```python
from build123d import *

# Parameters (mm, degrees)
F0_R     = 3.1
F1_DEPTH = 10
F2_DEPTH = 1.5
F3_W     = 10
F3_H     = 2
F4_DEPTH = 11.501


# Not quite as in the source:
# - a feature names something its author has since deleted; it is built from what else it names


with BuildPart() as f1:
    # F0 (on Top) → F1 (new body, symmetric)
    with BuildSketch(Plane.XY):
        Circle(F0_R)
    extrude(amount=F1_DEPTH, both=True)

    # F0 (on Top) → F2 (join, symmetric)
    with BuildSketch(Plane.XY):
        with BuildLine():
            ThreePointArc((1.6906574466, -9.8560477575), (7.6454749514, -6.4456739576), (10, 0))
            ThreePointArc((10, 0), (7.6454749525, 6.4456739563), (1.6906574499, 9.8560477569))
            ThreePointArc((1.6906574499, 9.8560477569), (-10, 1.7e-09), (1.6906574466, -9.8560477575))
        make_face()
        Circle(F0_R, mode=Mode.SUBTRACT)
        with BuildLine():
            ThreePointArc((1.6906574499, 9.8560477569), (7.6454749525, 6.4456739563), (10, 0))
            ThreePointArc((10, 0), (7.6454749514, -6.4456739576), (1.6906574466, -9.8560477575))
            Line((1.6906574466, -9.8560477575), (30, -5))
            Line((30, -5), (30, 5))
            Line((30, 5), (1.6906574499, 9.8560477569))
        make_face()
    extrude(amount=F2_DEPTH, both=True)

    # F3 (on face) → F4 (cut, through all)
    with BuildSketch(Plane.XY.offset(1.5)):
        with Locations((25, 0)):
            Rectangle(F3_W, F3_H)
    extrude(amount=-F4_DEPTH, mode=Mode.SUBTRACT)


solid = f1.part
```
Source: CAD feature listing. Evaluate the final solid. Frame: model axes, mm. A direction names the side the tool comes from. Coordinates: 2 decimals unless noted, no trailing zeros. Loops run counter-clockwise (first coordinate to the right, second up) from the corner with the lowest first, then second, coordinate; pieces in that order, holes last. Notation, with made-up numbers: (48.5, 31) -> (107.5, 31) arc R21 cw to (107.5, 61) -> close; hole circle Ø9 at (31, 12). An arc over 180 degrees is marked (long way). One line per item, written item: value. Start each with the question number.
Q1. Set-up query: faces 1 (the face through (1.43, -2.75, 5.81)), 2 (the face through (25, 1, 0)), 3 (the face through (1.43, -2.75, -5.69)). Return all of +Z, -Z, +X, -X, +Y, -Y with unobstructed straight access to the full face (end or side cutting, diameter ignored); none if empty.
Q2. Line query: line 1 along Z through (x, y) = (17.5, -5.5); line 2 along Y through (x, z) = (2.5, 3.5); line 3 along X through (y, z) = (0.75, -6). Output: solid intervals per line, ascending.
Q3. Contact query for flat-ended pins moving along their axis: P1, Ø1.5, axis at x = -4.5, z = 0.5, coming from the -Y side; P2, Ø6, axis at x = 11, y = 0.5, coming from the -Z side; P3, Ø3.5, axis at x = 25.5, z = 0.5, coming from the +Y side. Output: stop coordinate, or through.
Q4. Section query B-B, the plane z = 0.25. Return the cut outline in (x, y), and give its area (3 significant figures).
Q5. Mould query, pull axis Y, two halves, no side actions, for faces 4 (the face through (16, 7.4, 0)), 5 (the face through (0, 0, -10)), 6 (the face through (20, 0, 0)). Classes: pulls with the +Y half, pulls with the -Y half, needs draft (parallel to the pull), parting line crosses it, or undercut.
Q6. Section query A-A, the plane x = 21.5. Return the cut outline in (y, z).
Q7. Section query C-C, the plane y = 0. Return the cut outline in (x, z), and give its area (3 significant figures).
Q8. Section query D-D, the plane x = -1. Return the cut outline in (y, z), and give its area (3 significant figures).
Results:
1. face 1: +Z
1. face 2: +Z, -Z, +X
1. face 3: -Z
2. line 1: -1.5 to 1.5
2. line 2: -1.83 to 1.83
2. line 3: -3.01 to 3.01
3. P1: y = -9.27
3. P2: z = -1.5
3. P3: y = 6.07
4. outline: (1.69, -9.86) -> (30, -5) -> (30, -1) -> (20, -1) -> (20, 1) -> (30, 1) -> (30, 5) -> (1.69, 9.86) arc R10 ccw (long way) to start
4. area: 591 mm^2
5. face 4: pulls with the +Y half
5. face 5: needs draft
5. face 6: undercut
6. outline: (-6.46, -1.5) -> (-1, -1.5) -> (-1, 1.5) -> (-6.46, 1.5) -> close; (1, -1.5) -> (6.46, -1.5) -> (6.46, 1.5) -> (1, 1.5) -> close
7. outline: (-10, -1.5) -> (-3.1, -1.5) -> (-3.1, -10) -> (3.1, -10) -> (3.1, -1.5) -> (20, -1.5) -> (20, 1.5) -> (3.1, 1.5) -> (3.1, 10) -> (-3.1, 10) -> (-3.1, 1.5) -> (-10, 1.5) -> close
7. area: 195 mm^2
8. outline: (-9.95, -1.5) -> (-2.93, -1.5) -> (-2.93, -10) -> (2.93, -10) -> (2.93, -1.5) -> (9.95, -1.5) -> (9.95, 1.5) -> (2.93, 1.5) -> (2.93, 10) -> (-2.93, 10) -> (-2.93, 1.5) -> (-9.95, 1.5) -> close
8. area: 159 mm^2
